from build123d import *

# Parameters (mm, degrees)
SKETCH4_W           = 62.83623107
SKETCH4_H           = 84.722256574
BOSS_EXTRUDE2_DEPTH = 50
CUT_EXTRUDE2_DEPTH  = 80
CUT_EXTRUDE3_DEPTH  = 80
CUT_EXTRUDE5_DEPTH  = 80
CUT_EXTRUDE6_DEPTH  = 3
CUT_EXTRUDE8_DEPTH  = 80
CUT_EXTRUDE9_DEPTH  = 80
SKETCH11_W          = 5.870888161
SKETCH11_H          = 1.865764547
BOSS_EXTRUDE3_DEPTH = 20
SCALE1_SCALE        = 0.5
SCALE2_SCALE        = 0.4
SCALE3_SCALE        = 0.5
SCALE5_SCALE        = 4
SKETCH13_R          = 1.221118876
BOSS_EXTRUDE4_DEPTH = 2


with BuildPart() as part:
    # Sketch4 → Boss-Extrude2 (new body)
    with BuildSketch(Plane.XY):
        Rectangle(SKETCH4_W, SKETCH4_H)
    extrude(amount=BOSS_EXTRUDE2_DEPTH)

    # Sketch5 → Cut-Extrude2 (cut)
    with BuildSketch(Plane(origin=(31.418115535, 0, 0), x_dir=(0, 0, -1), z_dir=(1, 0, 0))):
        Polygon((-31.846034257, 38.728174008), (-31.846034257, 42.361128287), (-50, 42.361128287), (-50, -42.361128287), (-30.898434646, -42.361128287), (-30.898434646, -37.982426726), (-46.322270236, 2.38891709), align=None)
    extrude(amount=-CUT_EXTRUDE2_DEPTH, mode=Mode.SUBTRACT)

    # Sketch6 → Cut-Extrude3 (cut)
    with BuildSketch(Plane(origin=(31.418115535, 0, 0), x_dir=(0, 0, -1), z_dir=(1, 0, 0))):
        Polygon((-29.655383969, 42.361128287), (-29.655383969, 38.722554473), (-8.776416022, 3.750158878), (-28.328453067, -38.117745), (-28.328453067, -42.361128287), (-27.677514405, -46.625913761), (16.839811583, -52.045359618), (10.267667228, 27.190343951), (3.73953172, 54.484047391), align=None)
    extrude(amount=-CUT_EXTRUDE3_DEPTH, mode=Mode.SUBTRACT)

    # Sketch7 → Cut-Extrude5 (cut)
    with BuildSketch(Plane.ZY.offset(31.418115535)):
        with BuildLine():
            ThreePointArc((13.228873585, 11.208051798), (10.417703783, 4.563945687), (11.71087014, -2.533556863))
            ThreePointArc((11.71087014, -2.533556863), (0.747619784, 5.632177302), (13.228873585, 11.208051798))
        make_face()
    extrude(amount=-CUT_EXTRUDE5_DEPTH, mode=Mode.SUBTRACT)

    # Sketch8 → Cut-Extrude6 (cut)
    with BuildSketch(Plane(origin=(31.418115535, 0, 0), x_dir=(0, 0, -1), z_dir=(1, 0, 0))):
        Polygon((-30.111598921, 36.817435747), (-42.735074125, 2.19595341), (-30.111598921, -36.694083179), (-29.289064541, -37.07820135), (-12.845557678, 2.19595341), align=None)
    extrude(amount=-CUT_EXTRUDE6_DEPTH, mode=Mode.SUBTRACT)

    # Sketch9 → Cut-Extrude8 (cut)
    with BuildSketch(Plane(origin=(0, 0, 29.655383969), x_dir=(-1, 0, 0), z_dir=(0, 0, -1))):
        Polygon((19.869908303, 42.361128287), (19.869908303, 38.722554473), (19.869908303, 5.586987563), (19.869908303, -4.186945454), (19.869908303, -38.208459621), (19.869908303, -42.059759196), (19.869908303, -47.026854784), (41.256673117, -49.585938288), (42.081255469, -21.197702537), (42.081255469, 12.428184914), (37.482224788, 37.513066745), (31.418115535, 49.4837873), align=None)
    extrude(amount=-CUT_EXTRUDE8_DEPTH, mode=Mode.SUBTRACT)

    # Sketch10 → Cut-Extrude9 (cut)
    with BuildSketch(Plane(origin=(0, -2.877407212, 4.819674209), x_dir=(-1, 0, 0), z_dir=(0, 0.5126085745439567, -0.8586224136976701))):
        Polygon((19.869908303, 48.44965729), (25.693686727, -39.803296282), (32.448126733, -43.444815965), (49.802642339, -43.444815965), (32.448126733, 57.840856492), align=None)
    extrude(amount=-CUT_EXTRUDE9_DEPTH, mode=Mode.SUBTRACT)

    # Sketch11 → Boss-Extrude3 (add)
    with BuildSketch(Plane(origin=(0, 42.361128287, 0), x_dir=(1, 0, 0), z_dir=(0, 1, 0))):
        with Locations((4.437413085, -30.588266243)):
            Rectangle(SKETCH11_W, SKETCH11_H)
    extrude(amount=BOSS_EXTRUDE3_DEPTH)


with BuildPart() as part_1:
    # Scale1: scaled about (4.044501914, 0.935318094, 28.406526913)
    add(part.part.scale(SCALE1_SCALE).moved(Location((2.022250957, 0.467659047, 14.203263457))))


with BuildPart() as part_2:
    # Scale2: scaled about (4.044501914, 0.935318094, 28.406526913)
    add(part_1.part.scale(SCALE2_SCALE).moved(Location((2.426701148, 0.561190856, 17.043916148))))


with BuildPart() as part_3:
    # Scale3: scaled about (4.044501914, 0.935318094, 28.406526913)
    add(part_2.part.scale(SCALE3_SCALE).moved(Location((2.022250957, 0.467659047, 14.203263457))))


with BuildPart() as part_4:
    # Scale5: scaled about (4.044501914, 0.935318094, 28.406526913)
    add(part_3.part.scale(SCALE5_SCALE).moved(Location((-12.133505742, -2.805954282, -85.219580739))))


with BuildPart() as boss_extrude4_tool:
    # Sketch13 → Boss-Extrude4 (new body)
    with BuildSketch(Plane(origin=(0, -16.38326151, 0), x_dir=(-1, 0, 0), z_dir=(0, -1, 0))):
        with Locations(Location((-4.797778916, -28.817556161, 0), (0, 0, 331.33607571))):
            Circle(SKETCH13_R)
    extrude(amount=BOSS_EXTRUDE4_DEPTH)


with BuildPart() as part_5:
    add(part_4.part)


with BuildPart() as part_6:
    # Boss-Extrude4: joined with boss_extrude4_tool
    add(part_5.part.fuse(boss_extrude4_tool.part, tol=0.00001))


solid = part_6.part
Verification items for the finished model (mm, model axes). A direction names the side the tool comes from. Give positions to 0.01 mm unless a question says otherwise; leave off trailing zeros. Order: outer loops, then holes, each group sorted by start corner. A loop starts at its lowest first (then second) coordinate and runs counter-clockwise, first axis right, second up. Notation, with made-up numbers: (84, -13) -> (113, -13) arc R25 ccw to (113, 24) -> close; hole circle Ø10 at (63, 34.25). An arc over 180 degrees is marked (long way). Answer as CSV lines item,"result".
Q1. Scan lines: probe 1 along X at (y, z) = (8, 29); probe 2 along Y at (x, z) = (7.75, 29.25); probe 3 along Z at (x, y) = (11.25, -14). Record each from-to range of solid material in increasing order.
Solutions:
probe 1,"x = -5.52 to 13.79"
probe 2,"y = -16.38 to 17.51"
probe 3,"z = 28.05 to 29.64"
Q2. Sectioned sample at A-A on x = 10.25. Record the cut outline in (y, z), plus the area to 3 significant figures.
Solutions:
outline,"(-16.38, 28.38) -> (-14.69, 28.38) -> (-0.15, 21.59) arc R5.04 ccw to (3.73, 21.55) -> (16.05, 28.91) -> (17.51, 28.91) -> (17.51, 29.78) -> (16.05, 29.78) -> (1.52, 35.57) -> (-14.63, 29.4) -> (-16.38, 29.4) -> close"
area,"248 mm²"
Q3. Sectioned sample at D-D on y = -7. Record the cut outline in (x, z), plus the area to 3 significant figures.
Solutions:
outline,"(-6.97, 24.79) -> (14.99, 24.79) -> (14.99, 25.72) -> (13.79, 25.72) -> (13.79, 31.4) -> (14.99, 31.4) -> (14.99, 32.32) -> (-5.52, 32.32) -> (-5.52, 28.91) -> (-6.83, 28.91) -> close"
area,"153 mm²"
Q4. Access from +Z, -Z, +X, -X, +Y, -Y to the whole of each face (thin tool, end or side, straight path). Record for faces 4 (the flat face through (5, 17, 29.782)), 5 (the flat face through (5, 19, 28.906)), 6 (the cylindrical face through (4.357, -17.369, 27.679)), 7 (the flat face through (14.4, -6.23, 31.65)), 8 (the flat face through (-5.521, 1, 31)).
Solutions:
face 4,"+Z, +X, -X, +Y"
face 5,"-Z, +X, -X, +Y"
face 6,"-Y"
face 7,"+X"
face 8,"+Z, -X, +Y, -Y"
Q5. Depth check by flat-ended pin: pin 1 (5.5 mm diameter, centred on y = 5.5, z = 32, fed in from -X); pin 2 (6 mm diameter, centred on x = -5, z = 32, fed in from +Y); pin 3 (1.2 mm diameter, centred on x = 3.5, y = 17, fed in from +Z); pin 4 (6 mm diameter, centred on x = 4, z = 27, fed in from -Y). Enter the tip coordinate at first touch or a pass-through.
Solutions:
pin 1,"stops at x = -5.52"
pin 2,"stops at y = 17.51"
pin 3,"stops at z = 29.78"
pin 4,"stops at y = -18.38"
Q6. Release check for a two-part mould opening along Y. For faces 1 (the flat face through (4, 21, 29.652)), 2 (the flat face through (14.4, -6.53, 25.52)), 3 (the flat face through (4.41, 9.98, 25.28)) record: +Y half, -Y half, draft (parallel to the pull), parting line (faces both ways), or undercut.
Solutions:
face 1,"draft"
face 2,"undercut"
face 3,"+Y half"
Q7. Sectioned sample at B-B on y = 14.5. Record the cut outline in (x, z).
Solutions:
outline,"(-5.64, 27.98) -> (14.99, 27.98) -> (14.99, 28.7) -> (13.79, 28.7) -> (13.79, 29.38) -> (14.99, 29.38) -> (14.99, 30.4) -> (-5.52, 30.4) -> (-5.52, 28.91) -> (-5.61, 28.91) -> close"
Q8. Sectioned sample at C-C on z = 33.25. Record the cut outline in (x, y).
Solutions:
outline,"(-5.52, -4.56) -> (14.99, -4.56) -> (14.99, -1.3) -> (13.79, -1.3) -> (13.79, 3.87) -> (14.99, 3.87) -> (14.99, 7.35) -> (-5.52, 7.35) -> close"
